```python
from build123d import *

# Parameters (mm, degrees)
SKETCH_1_W                  = 320
SKETCH_1_H                  = 200
EXTRUDE_1_DEPTH             = 287
SKETCH_2_R                  = 11
CUT_EXTRUDE_1_DEPTH         = 475.098091116
PATTERN_LINEAR_1_COUNT      = 4
PATTERN_LINEAR_1_PITCH      = 80
PATTERN_LINEAR_1_COUNT_DIR2 = 2
PATTERN_LINEAR_1_PITCH_DIR2 = 110
SKETCH_6_W                  = 261
SKETCH_6_H                  = 93.5
CUT_EXTRUDE_3_DEPTH         = 475.098091116


with BuildPart() as part:
    # 草图1 → 拉伸1 (new body)
    with BuildSketch(Plane.XY):
        with Locations((160, 100)):
            Rectangle(SKETCH_1_W, SKETCH_1_H)
    extrude(amount=EXTRUDE_1_DEPTH)

    # 草图2 → 切除-拉伸1 (cut, through all)
    with BuildSketch(Plane.XY.offset(287)):
        with Locations((40, 45)):
            Circle(SKETCH_2_R)
    cut_extrude_1 = extrude(amount=-CUT_EXTRUDE_1_DEPTH, mode=Mode.SUBTRACT)

    # 阵列(线性)1: Cut-Extrude 1 4 × 2
    with Locations(*[(i * PATTERN_LINEAR_1_PITCH, j * PATTERN_LINEAR_1_PITCH_DIR2, 0) for i in range(PATTERN_LINEAR_1_COUNT) for j in range(PATTERN_LINEAR_1_COUNT_DIR2) if (i, j) != (0, 0)]):
        add(cut_extrude_1, mode=Mode.SUBTRACT)

    # 草图6 → 切除-拉伸3 (cut, through all)
    with BuildSketch(Plane.ZY):
        with Locations((143.5, 153.25)):
            Rectangle(SKETCH_6_W, SKETCH_6_H)
        with Locations((143.5, 46.75)):
            Rectangle(SKETCH_6_W, SKETCH_6_H)
    extrude(amount=-CUT_EXTRUDE_3_DEPTH, mode=Mode.SUBTRACT)


solid = part.part
```
Model file for the job. Use its own axes, mm. A direction names the side the tool comes from. Round coordinates to 2 decimals unless told otherwise and drop trailing zeros. Order: outer loops, then holes, each group sorted by start corner. A loop starts at its lowest first (then second) coordinate and runs counter-clockwise, first axis right, second up. Notation, with made-up numbers: M -18,47 L -3,47 A28 ccw -3,70 Z; hole C 19,-37.5 d7. An arc over 180 degrees is marked long. Use CSV: the item, a comma, the result in double quotes.
Item 1: Pin check, flat tips, straight feed: pin 1 (13 mm diameter, centred on x = 40, y = 155, fed in from +Z); pin 2 (1 mm diameter, centred on x = 243.5, z = 148.5, fed in from -Y); pin 3 (12 mm diameter, centred on x = 217, z = 39.5, fed in from +Y). Stop position of each tip, or through.
Worked answers:
pin 1,"through"
pin 2,"y = 93.5"
pin 3,"y = 106.5"
Item 2: Pull direction Y, two halves, no side cores. Call faces 4 (the face through (158, 101, 287)), 5 (the face through (191.89, 162.43, 280.59)), 6 (the face through (158, 200, 280)), 7 (the face through (158, 0, 6)): released by +Y, released by -Y, zero draft, split by the parting line, or undercut.
Worked answers:
face 4,"zero draft"
face 5,"undercut"
face 6,"released by +Y"
face 7,"released by -Y"
Item 3: Saw through at A-A (x = 76). List the corners of the cut face in (y, z).
Worked answers:
outline,"M 0,0 L 200,0 L 200,13 L 106.5,13 L 106.5,274 L 200,274 L 200,287 L 0,287 L 0,274 L 93.5,274 L 93.5,13 L 0,13 Z"
Item 4: Probe probe 1 along Y at (x, z) = (120, 284); probe 2 along Z at (x, y) = (238, 118); probe 3 along Y at (x, z) = (138, 88.5). List the from-to ranges inside material, lowest first.
Worked answers:
probe 1,"0 to 34, 56 to 144, 166 to 200"
probe 2,"0 to 13, 274 to 287"
probe 3,"93.5 to 106.5"
Item 5: Saw through at B-B (y = 181). List the corners of the cut face in (x, z), plus the area to 3 significant figures.
Worked answers:
outline,"M 0,0 L 320,0 L 320,13 L 0,13 Z; M 0,274 L 320,274 L 320,287 L 0,287 Z"
area,"8,320 mm²"
Item 6: Saw through at D-D (y = 45). State how many separate pieces and enclosed holes the cut face has, plus the area to 3 significant figures.
Worked answers:
separate pieces,"10"
enclosed holes,"0"
area,"6,030 mm²"
Item 7: Which spindle directions (+Z, -Z, +X, -X, +Y, -Y) get a long thin tool onto all of the face, cutting with end or side? Do faces 1 (the face through (158, 46, 13)), 2 (the face through (269, 155, 281)), 3 (the face through (158, 153, 274)). Say none if no direction does.
Worked answers:
face 1,"+X, -X, -Y"
face 2,"+Z, -Z"
face 3,"+X, -X, +Y"
Item 8: Saw through at C-C (x = 120). List the corners of the cut face in (y, z), plus the area to 3 significant figures.
Worked answers:
outline,"M 0,0 L 34,0 L 34,13 L 0,13 Z; M 0,274 L 34,274 L 34,287 L 0,287 Z; M 56,0 L 144,0 L 144,13 L 106.5,13 L 106.5,274 L 144,274 L 144,287 L 56,287 L 56,274 L 93.5,274 L 93.5,13 L 56,13 Z; M 166,0 L 200,0 L 200,13 L 166,13 Z; M 166,274 L 200,274 L 200,287 L 166,287 Z"
area,"7,450 mm²"
